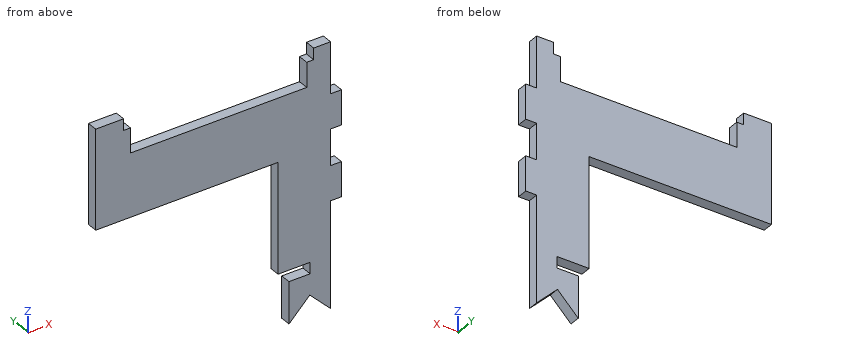
```python
from build123d import *

# Parameters (mm, degrees)
BOSS_EXTRUDE1_DEPTH = 3
SKETCH6_W           = 3.2
SKETCH6_H           = 30.2
SKETCH6_H_2         = 10.2
CUT_EXTRUDE3_DEPTH  = 4


with BuildPart() as part:
    # Sketch1 → Boss-Extrude1 (new body)
    with BuildSketch(Plane(origin=(0, 0, 0), x_dir=(1, 0, 0), z_dir=(0, 1, 0))):
        Polygon((-34.872217102, 0), (34.872217102, 0), (34.872217102, 75), (31.872217102, 75), (25.872217102, 69), (19.872217102, 75), (16.872217102, 75), (16.872217102, 28.75), (-34.872217102, 28.75), align=None)
    extrude(amount=BOSS_EXTRUDE1_DEPTH)

    # Sketch6 → Cut-Extrude3 (cut, through all)
    with BuildSketch(Plane(origin=(0, 0, 0), x_dir=(1, 0, 0), z_dir=(0, 1, 0))):
        with Locations((33.372217102, 60)):
            Rectangle(SKETCH6_W, SKETCH6_H)
        with Locations((33.372217102, 30)):
            Rectangle(SKETCH6_W, SKETCH6_H_2)
        Polygon((25.972217102, 63.1), (19.972217102, 63.1), (19.972217102, 75.1), (16.772217102, 75.1), (16.772217102, 59.9), (25.972217102, 59.9), align=None)
        Polygon((34.972217102, -0.1), (34.972217102, 15.1), (31.772217102, 15.1), (31.772217102, 0.6), (26.972217102, 0.6), (26.972217102, 3.85), (25.008726501, 3.85), (25.008726501, 10.85), (-25.008726501, 10.85), (-25.008726501, 3.85), (-26.972217102, 3.85), (-26.972217102, 0.6), (-34.972217102, 0.6), (-34.972217102, -0.1), align=None)
    extrude(amount=CUT_EXTRUDE3_DEPTH, mode=Mode.SUBTRACT)


solid = part.part
```
Model file for the job. Use its own axes, mm. Give positions to 0.01 mm unless a question says otherwise; leave off trailing zeros. Order: outer loops, then holes, each group sorted by start corner. A loop starts at its lowest first (then second) coordinate and runs counter-clockwise, first axis right, second up.
1) Saw through at C-C, the plane z = -64. Write the cut outline in (x, y), then the cut area to 3 significant figures.
2) Pin check, flat tips, straight feed: pin 1 (0.9 mm diameter, centred on y = 1, z = -48, fed in from -X); pin 2 (1.6 mm diameter, centred on x = 26, y = 1.5, fed in from +Z); pin 3 (0.9 mm diameter, centred on y = 2, z = -2.5, fed in from +X); pin 4 (1.5 mm diameter, centred on x = 17, z = -60.5, fed in from +Y). Stop position of each tip, or through.
3) Wall check: probe 1 along X at (y, z) = (2.2, -4); probe 2 along Z at (x, y) = (6, 2.75); probe 3 along X at (y, z) = (0.6, -55). Give the ranges that are in metal, low to high.
4) Saw through at B-B, the plane y = 0.6. Write the cut outline in (x, z), then the cut area to 3 significant figures.
5) Saw through at D-D, the plane x = -11.5. Write the cut outline in (y, z).
6) Saw through at A-A, the plane x = 21. Write the cut outline in (y, z), then the cut area to 3 significant figures.
Computed:
1. outline: (19.97, 0) - (31.77, 0) - (31.77, 3) - (19.97, 3) - close
1. area: 35.4 mm2
2. pin 1: stops at x = 16.87
2. pin 2: stops at z = -3.85
2. pin 3: stops at x = 31.77
2. pin 4: stops at y = 3
3. probe 1: x = -34.87 to -25.01, 25.01 to 31.77
3. probe 2: z = -28.75 to -10.85
3. probe 3: x = 16.87 to 31.77
4. outline: (-34.87, -28.75) - (16.87, -28.75) - (16.87, -59.9) - (25.97, -59.9) - (25.97, -63.1) - (19.97, -63.1) - (19.97, -74.9) - (25.87, -69) - (31.77, -74.9) - (31.77, -44.9) - (34.87, -44.9) - (34.87, -35.1) - (31.77, -35.1) - (31.77, -24.9) - (34.87, -24.9) - (34.87, -15.1) - (31.77, -15.1) - (31.77, -0.6) - (26.97, -0.6) - (26.97, -3.85) - (25.01, -3.85) - (25.01, -10.85) - (-25.01, -10.85) - (-25.01, -3.85) - (-26.97, -3.85) - (-26.97, -0.6) - (-34.87, -0.6) - close
4. area: 2,000 mm2
5. outline: (0, -28.75) - (3, -28.75) - (3, -10.85) - (0, -10.85) - close
6. outline: (0, -73.87) - (3, -73.87) - (3, -63.1) - (0, -63.1) - close; (0, -59.9) - (3, -59.9) - (3, -10.85) - (0, -10.85) - close
6. area: 179 mm2
